The model under review builds one solid part; all positions refer to its coordinate system, in mm. A direction names the side the tool comes from. Coordinates: 2 decimals unless noted, no trailing zeros. Loops run counter-clockwise (first coordinate to the right, second up) from the corner with the lowest first, then second, coordinate; pieces in that order, holes last. Notation, with made-up numbers: (-32, -40) - (-4, -40) arc R19 cw to (-4, -35) - close; hole circle Ø8 at (64.25, -25). An arc over 180 degrees is marked (long way). One line per item, written item: value. Start each with the question number.
1. For faces 4 (the face through (13, 4, 0)), 5 (the face through (13, -3, 1)), list the 3-axis set-ups (+Z, -Z, +X, -X, +Y, -Y) from which the entire face can be reached by the end or side of a thin tool; tool diameter is ignored.
2. To check wall thickness, follow line 1 (Y direction, x = 26, z = 1.9); line 2 (X direction, y = -0.5, z = 2.6); line 3 (X direction, y = 0.75, z = 0.9). State the ranges of each line that lie inside material, in increasing order.
3. We need section D-D, the plane y = -2.25. Give the boundary of the cut face in (x, z).
4. We need section C-C, the plane x = -2. Give the boundary of the cut face in (y, z).
5. We need section A-A, the plane y = 0. Give the boundary of the cut face in (x, z).
6. Mouldability with a two-part tool opening along Y and no side actions: class faces 1 (the face through (13, 6, 1)), 2 (the face through (7, 0, 1)), 3 (the face through (-6, 0, 1)) as +Y half, -Y half, draft (parallel to the pull), parting line (faces both ways), or undercut.
7. We need section B-B, the plane z = 2.2. Give the boundary of the cut face in (x, y).
from build123d import *

# Parameters (mm, degrees)
SKETCH_2_R      = 3
EXTRUDE_1_DEPTH = 3


with BuildPart() as part:
    # 草图2 → 凸台-拉伸1 (new body)
    with BuildSketch(Plane.XY):
        with BuildLine():
            Line((0, 6), (26, 6))
            ThreePointArc((26, 6), (32, 0), (26, -6))
            Line((26, -6), (0, -6))
            ThreePointArc((0, -6), (-6, 0), (0, 6))
        make_face()
        Circle(SKETCH_2_R, mode=Mode.SUBTRACT)
        with Locations((26, 0)):
            Circle(SKETCH_2_R, mode=Mode.SUBTRACT)
        with BuildLine():
            Line((10, 3), (16, 3))
            ThreePointArc((16, 3), (19, 0), (16, -3))
            Line((16, -3), (10, -3))
            ThreePointArc((10, -3), (7, 0), (10, 3))
        make_face(mode=Mode.SUBTRACT)
    extrude(amount=EXTRUDE_1_DEPTH)


solid = part.part
Findings below:
1. face 4: -Z, +X, -X, +Y, -Y
1. face 5: +Z, -Z
2. line 1: -6 to -3, 3 to 6
2. line 2: -5.98 to -2.96, 2.96 to 7.04, 18.96 to 23.04, 28.96 to 31.98
2. line 3: -5.95 to -2.9, 2.9 to 7.1, 18.9 to 23.1, 28.9 to 31.95
3. outline: (-5.56, 0) - (-1.98, 0) - (-1.98, 3) - (-5.56, 3) - close; (1.98, 0) - (8.02, 0) - (8.02, 3) - (1.98, 3) - close; (17.98, 0) - (24.02, 0) - (24.02, 3) - (17.98, 3) - close; (27.98, 0) - (31.56, 0) - (31.56, 3) - (27.98, 3) - close
4. outline: (-5.66, 0) - (-2.24, 0) - (-2.24, 3) - (-5.66, 3) - close; (2.24, 0) - (5.66, 0) - (5.66, 3) - (2.24, 3) - close
5. outline: (-6, 0) - (-3, 0) - (-3, 3) - (-6, 3) - close; (3, 0) - (7, 0) - (7, 3) - (3, 3) - close; (19, 0) - (23, 0) - (23, 3) - (19, 3) - close; (29, 0) - (32, 0) - (32, 3) - (29, 3) - close
6. face 1: +Y half
6. face 2: undercut
6. face 3: parting line
7. outline: (0, -6) - (26, -6) arc R6 ccw to (26, 6) - (0, 6) arc R6 ccw to start; hole circle Ø6 at (0, 0); hole (10, -3) - (16, -3) arc R3 ccw to (16, 3) - (10, 3) arc R3 ccw to start; hole circle Ø6 at (26, 0)
